from build123d import *

# Parameters (mm, degrees)
EXTRUDE_THIN2_DEPTH = 5
CUT_EXTRUDE1_REACH  = 21.502
SKETCH2_R           = 1


with BuildPart() as part:
    # Sketch1 → Extrude-Thin2 (new body)
    with BuildSketch(Plane.XY):
        with BuildLine():
            Line((8.683836794, 7.227072274), (11.620904097, 8.922788872))
            ThreePointArc((11.620904097, 8.922788872), (11.983877658, 9.856173835), (11.151179503, 10.412564954))
            Line((11.151179503, 10.412564954), (6.74601462, 10.027162966))
            ThreePointArc((6.74601462, 10.027162966), (6.467656906, 9.942060472), (6.247978783, 9.751097193))
            Line((6.247978783, 9.751097193), (-0.496472901, 0.800907512))
            ThreePointArc((-0.496472901, 0.800907512), (-0.544622327, 0.276901093), (-0.097155146, 0))
            Line((-0.097155146, 0), (0, 0))
            Line((0, 0), (15, 0))
            Line((15, 0), (15, -1))
            Line((15, -1), (0, -1))
            Line((0, -1), (-0.097155146, -1))
            ThreePointArc((-0.097155146, -1), (-1.439556688, -0.16929672), (-1.295108411, 1.402722535))
            Line((-1.295108411, 1.402722535), (5.449343273, 10.352912216))
            ThreePointArc((5.449343273, 10.352912216), (5.982847286, 10.816680179), (6.658858877, 11.023357664))
            Line((6.658858877, 11.023357664), (11.064023761, 11.408759652))
            ThreePointArc((11.064023761, 11.408759652), (12.937594609, 10.156879635), (12.120904097, 8.056763469))
            Line((12.120904097, 8.056763469), (9.183836794, 6.36104687))
            Line((9.183836794, 6.36104687), (8.683836794, 7.227072274))
        make_face()
    extrude(amount=EXTRUDE_THIN2_DEPTH)

    # Sketch2 → Cut-Extrude1 (cut, up to next)
    with BuildSketch(Plane(origin=(0, 0, 0), x_dir=(1, 0, 0), z_dir=(0, 1, 0)), mode=Mode.PRIVATE) as cut_extrude1_sk1:
        with Locations(Location((7.451422427, -2.5, 0), (0, 0, 270))):
            Circle(SKETCH2_R)
    cut_extrude1_tool1 = extrude(cut_extrude1_sk1.sketch, amount=-CUT_EXTRUDE1_REACH, mode=Mode.PRIVATE) & part.part
    add(cut_extrude1_tool1.solids().sort_by_distance((7.451422, 0, 2.5))[0], mode=Mode.SUBTRACT)


solid = part.part
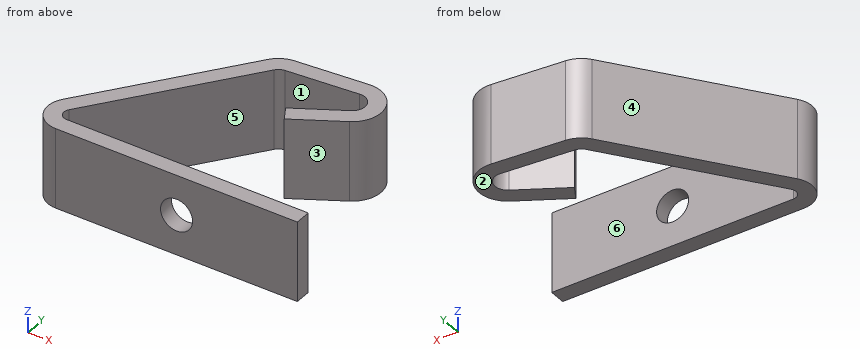
Model file for the job. Use its own axes, mm. Face numbers are marked on the shaded views. A direction names the side the tool comes from. Give positions to 0.01 mm unless a question says otherwise; leave off trailing zeros. Loops run counter-clockwise (first coordinate to the right, second up) from the corner with the lowest first, then second, coordinate; pieces in that order, holes last. Notation, with made-up numbers: (42.5, 74.25) -> (93.5, 74.25) arc R22 cw to (93.5, 82.25) -> close; hole circle Ø7 at (33.25, -28.75). An arc over 180 degrees is marked (long way). Use a Markdown table: item, result. Add a question column.
(1) Mould opens along X. For the marked faces 1, 2 and 3 say: +X half, -X half, draft (parallel to the pull), parting line (faces both ways), or undercut.
(2) Slice it at A-A on z = 2.5. List the corners of the cut face in (x, y), and give its area (3 significant figures).
(3) Wall check: line 1 along Y through (x, z) = (10.5, 4.4); line 2 along Y through (x, z) = (11.25, 4.05); line 3 along X through (y, z) = (-0.4, 2.5). Give the ranges that are in metal, low to high.
(4) Slice it at C-C on x = 1.25. List the corners of the cut face in (y, z).
(5) Slice it at B-B on y = 6.75. List the corners of the cut face in (x, z), and give its area (3 significant figures).
(6) Drop flat-ended pins along their axis: pin 1 Ø1 at (x, z) = (8, 2.5) entering from +Y; pin 2 Ø3 at (y, z) = (8, 2) entering from +X; pin 3 Ø1.5 at (x, z) = (10, 2.5) entering from +Y. Give the stop position or say it passes through.
(7) Tool access for the marked faces 4, 5 and 6: list every direction of +Z, -Z, +X, -X, +Y, -Y with a clear straight run to the whole face (end or side of a thin tool).
(8) Slice it at D-D on y = 2.5. List the corners of the cut face in (x, z).
Filled sheet:
| question | item | result |
|---|---|---|
| 1 | face 1 | undercut |
| 1 | face 2 | draft |
| 1 | face 3 | +X half |
| 2 | outline | (-1.3, 1.4) arc R1.5 ccw to (-0.1, -1) -> (6.45, -1) -> (6.45, 0) -> (-0.1, 0) arc R0.5 cw to (-0.5, 0.8) -> (6.25, 9.75) arc R0.7 cw to (6.75, 10.03) -> (11.15, 10.41) arc R0.8 cw to (11.62, 8.92) -> (8.68, 7.23) -> (9.18, 6.36) -> (12.12, 8.06) arc R1.8 ccw to (11.06, 11.41) -> (6.66, 11.02) arc R1.7 ccw to (5.45, 10.35) -> close; (8.45, -1) -> (15, -1) -> (15, 0) -> (8.45, 0) -> close |
| 2 | area | 38.9 mm2 |
| 3 | line 1 | -1 to 0, 7.12 to 8.28, 10.36 to 11.36 |
| 3 | line 2 | -1 to 0, 7.55 to 8.71, 10.42 to 11.42 |
| 3 | line 3 | -1.3 to 6.45, 8.45 to 15 |
| 4 | outline | (-1, 0) -> (0, 0) -> (0, 5) -> (-1, 5) -> close; (3.12, 0) -> (4.78, 0) -> (4.78, 5) -> (3.12, 5) -> close |
| 5 | outline | (2.73, 0) -> (3.99, 0) -> (3.99, 5) -> (2.73, 5) -> close; (8.96, 0) -> (9.86, 0) -> (9.86, 5) -> (8.96, 5) -> close |
| 5 | area | 10.8 mm2 |
| 6 | pin 1 | y = 11.18 |
| 6 | pin 2 | x = 13.02 |
| 6 | pin 3 | y = 11.38 |
| 7 | face 4 | +Z, -Z, -X, +Y |
| 7 | face 5 | +Z, -Z |
| 7 | face 6 | +Z, -Z, +X |
| 8 | outline | (-0.47, 0) -> (0.78, 0) -> (0.78, 5) -> (-0.47, 5) -> close |
